from build123d import *

# Parameters (mm, degrees)
SKETCH1_R           = 3.1750000000000016
SKETCH1_R_2         = 3.174999999999998
SKETCH1_R_3         = 3.1749999999999976
BOSS_EXTRUDE1_DEPTH = 5.842
FILLET1_R           = 6.35
FILLET2_R           = 12.7
BOSS_EXTRUDE2_START = -5.842
SKETCH2_R           = 3.3749999999999933
BOSS_EXTRUDE2_DEPTH = 5.842
SKETCH3_R           = 3.174229815615873
CUT_EXTRUDE1_DEPTH  = 74.47150684282778
FILLET3_R           = 6.35
CUT_EXTRUDE2_DEPTH  = 74.47150698753184
FILLET4_R           = 6.35


with BuildPart() as part:
    # Sketch1 → Boss-Extrude1 (new body)
    with BuildSketch(Plane.XY):
        with BuildLine():
            Line((-19.735202783136515, 15.926469991088537), (-23.82219128055887, 21.14411855360569))
            ThreePointArc((-23.82219128055887, 21.14411855360569), (-23.43878883536159, 29.420896018239304), (-15.19702887852625, 30.27262100199607))
            Line((-15.19702887852625, 30.27262100199607), (-1.1351215821202347, 20.490721215283713))
            Line((-1.1351215821202347, 20.490721215283713), (26.98869301069201, 20.49072121528371))
            Line((26.98869301069201, 20.49072121528371), (42.6381003070978, 30.272621001996075))
            ThreePointArc((42.6381003070978, 30.272621001996075), (50.87986026393313, 29.42089601823929), (51.26326270913039, 21.14411855360571))
            Line((51.26326270913039, 21.14411855360571), (47.176274211707955, 15.926469991088574))
            Line((47.176274211707955, 15.926469991088574), (47.176274211707955, 5.491172866054349))
            Line((47.176274211707955, 5.491172866054349), (51.26326270913039, 0.27352430353700524))
            ThreePointArc((51.26326270913039, 0.27352430353700524), (52.26703524751068, -1.5710682312081294), (52.614285714285785, -3.6421785714286505))
            Line((52.614285714285785, -3.6421785714286505), (52.614285714285785, -37.659455709821316))
            Line((52.614285714285785, -37.659455709821316), (-25.173214285713918, -37.659455709821316))
            Line((-25.173214285713918, -37.659455709821316), (-25.173214285713925, -3.6421785714286505))
            ThreePointArc((-25.173214285713925, -3.6421785714286505), (-24.825963818939076, -1.5710682312081503), (-23.822191280558854, 0.27352430353699286))
            Line((-23.822191280558854, 0.27352430353699286), (-19.735202783136522, 5.491172866054132))
            Line((-19.735202783136522, 5.491172866054132), (-19.735202783136515, 15.926469991088537))
        make_face()
        with Locations((-18.823214285714226, 25.059821428571347)):
            Circle(SKETCH1_R, mode=Mode.SUBTRACT)
        with Locations((46.26428571428577, 25.059821428571347)):
            Circle(SKETCH1_R_2, mode=Mode.SUBTRACT)
        with Locations((46.26428571428577, -3.6421785714286505)):
            Circle(SKETCH1_R_3, mode=Mode.SUBTRACT)
        with Locations((-18.823214285713924, -3.6421785714286505)):
            Circle(SKETCH1_R, mode=Mode.SUBTRACT)
    extrude(amount=BOSS_EXTRUDE1_DEPTH)

    # Fillet1
    fillet1_edges = [part.edges().sort_by_distance(p)[0] for p in [
        (47.176274211707955, 15.926469991088574, 2.921),
        (47.176274211707955, 5.491172866054349, 2.921),
        (-19.735202783136522, 5.491172866054132, 2.921),
        (-19.735202783136515, 15.926469991088537, 2.921),
    ]]
    fillet(fillet1_edges, radius=FILLET1_R)

    # Fillet2
    fillet2_edges = [part.edges().sort_by_distance(p)[0] for p in [
        (-1.1351215821202347, 20.490721215283713, 2.921),
        (26.98869301069201, 20.49072121528371, 2.921),
    ]]
    fillet(fillet2_edges, radius=FILLET2_R)

    # Sketch2 → Boss-Extrude2 (add)
    # profile 1 of 2: a face of its own
    with BuildSketch(Plane.XY.offset(5.842).offset(BOSS_EXTRUDE2_START)):
        with BuildLine():
            Line((52.614285714285785, -22.564372384825948), (56.4647972168636, -22.564372384825948))
            ThreePointArc((56.4647972168636, -22.564372384825948), (62.8147972168636, -16.214372384825946), (56.4647972168636, -9.864372384825945))
            Line((56.4647972168636, -9.864372384825945), (51.94643033410118, -0.8074418077232544))
            ThreePointArc((51.94643033410118, -0.8074418077232544), (52.44506715095817, -2.186005219081439), (52.614285714285785, -3.6421785714286505))
            Line((52.614285714285785, -3.6421785714286505), (52.614285714285785, -11.165009933138013))
            Line((52.614285714285785, -11.165009933138013), (52.614285714285785, -21.26373483651388))
            Line((52.614285714285785, -21.26373483651388), (52.614285714285785, -22.564372384825948))
        make_face()
        with Locations((56.4647972168636, -16.214372384825946)):
            Circle(SKETCH2_R, mode=Mode.SUBTRACT)
    # profile 2 of 2: a face of its own
    with BuildSketch(Plane.XY.offset(5.842).offset(BOSS_EXTRUDE2_START)):
        with BuildLine():
            Line((-25.11442078188718, -2.7800760122689354), (-26.085202783136417, -9.864372384825948))
            ThreePointArc((-26.085202783136417, -9.864372384825948), (-32.43520278313642, -16.21437238482595), (-26.085202783136413, -22.56437238482595))
            Line((-26.085202783136417, -22.56437238482595), (-25.17321428571397, -22.56437238482595))
            Line((-25.17321428571397, -22.56437238482595), (-25.17321428571397, -22.49854114294895))
            Line((-25.173214285713975, -22.49854114294895), (-25.173214285713986, -19.254769053504887))
            ThreePointArc((-25.173214285713996, -19.254769053504887), (-29.25943259875229, -16.214372384825957), (-25.17321428571401, -13.173975716147009))
            Line((-25.173214285714007, -13.173975716147009), (-25.17321428571402, -9.930203626702937))
            Line((-25.17321428571402, -9.930203626702937), (-25.173214285714042, -3.6421785714286496))
            ThreePointArc((-25.173214285714042, -3.6421785714286496), (-25.158498859065922, -3.2101260576638357), (-25.11442078188718, -2.7800760122689354))
        make_face()
    extrude(amount=BOSS_EXTRUDE2_DEPTH)

    # Sketch3 → Cut-Extrude1 (cut, through all)
    with BuildSketch(Plane.XY.offset(5.842)):
        with Locations((-26.085202783136417, -16.21437238482595)):
            Circle(SKETCH3_R)
    extrude(amount=-CUT_EXTRUDE1_DEPTH, mode=Mode.SUBTRACT)

    # Fillet3
    fillet3_edges = [part.edges().sort_by_distance(p)[0] for p in [
        (56.4647972168636, -9.864372384825945, 2.921),
        (52.614285714285785, -22.564372384825948, 2.921),
        (-25.17321428571397, -22.56437238482595, 2.921),
        (-26.085202783136417, -9.864372384825948, 2.921),
    ]]
    fillet(fillet3_edges, radius=FILLET3_R)

    # Sketch4 → Cut-Extrude2 (cut, through all)
    with BuildSketch(Plane.XY.offset(5.842)):
        with BuildLine():
            Line((-25.173214285713918, -37.659455709821316), (-12.473214285713917, -37.659455709821316))
            Line((-12.473214285713917, -37.659455709821316), (-27.048811913081487, -23.185421123073148))
            ThreePointArc((-27.048811913081487, -23.185421123073148), (-25.66083613916725, -25.250928515915028), (-25.17321428571392, -27.691219987623278))
            Line((-25.17321428571392, -27.691219987623278), (-25.173214285713918, -37.659455709821316))
        make_face()
        with BuildLine():
            Line((54.888473112152276, -23.796663637650127), (38.326785714286075, -37.659455709821316))
            Line((38.326785714286075, -37.659455709821316), (52.614285714285785, -37.659455709821316))
            Line((52.614285714285785, -37.659455709821316), (52.614285714285785, -28.665981005853762))
            ThreePointArc((52.614285714285785, -28.665981005853762), (53.21085586664066, -25.97887382745055), (54.888473112152276, -23.796663637650127))
        make_face()
    extrude(amount=-CUT_EXTRUDE2_DEPTH, mode=Mode.SUBTRACT)

    # Fillet4
    fillet4_edges = [part.edges().sort_by_distance(p)[0] for p in [
        (-12.473214285713917, -37.659455709821316, 2.921),
        (38.326785714286075, -37.659455709821316, 2.921),
    ]]
    fillet(fillet4_edges, radius=FILLET4_R)


solid = part.part
CAD build for the part. Positions are in the model's coordinates, mm. A direction names the side the tool comes from. Give positions to 0.01 mm unless a question says otherwise; leave off trailing zeros. Loops run counter-clockwise (first coordinate to the right, second up) from the corner with the lowest first, then second, coordinate; pieces in that order, holes last. Notation, with made-up numbers: M -33.75,52.25 L -1.75,52.25 A22 ccw -1.75,86.25 Z; hole C 33,49 d3. An arc over 180 degrees is marked long. One line per question, with ' | ' between items. Start each with the question number.
1. Saw through at B-B on y = 27. Give the cut face in (x, z), plus the area to 3 significant figures.
2. Saw through at C-C on x = 16. Give the cut face in (y, z).
3. Saw through at D-D on z = 2.4. State how many separate pieces and enclosed holes the cut face has, plus the area to 3 significant figures.
4. Probe L1, parallel to X at y = -17, z = 4.1; L2, parallel to X at y = 25.5, z = 0.3; L3, parallel to Y at x = 59.5, z = 1.65. List the from-to ranges inside material, lowest first. Write a range as from..to.
5. Two-plate mould, pull along X, no slides. Class faces 6 (the face through (53.79, -18.27, 2.88)), 7 (the face through (47.514, 5.639, 2.962)), 8 (the face through (15, -3, 0)): pulls with the +X half, pulls with the -X half, needs draft (parallel to the pull), parting line crosses it, or undercut.
6. Saw through at A-A on y = -17.5. Give the cut face in (x, z), plus the area to 3 significant figures.
7. 3-axis set-ups, long thin cutter, end or side, ignore diameter. For faces 1 (the face through (47.6, -29.9, 3)), 2 (the face through (49.293, -2.688, 2.88)), 3 (the face through (-24.68, -1.19, 2.88)), 4 (the face through (49.88, 2.04, 2.88)), 5 (the face through (13, 20.491, 3)): which of +Z, -Z, +X, -X, +Y, -Y reach the whole face in a straight line?
8. Flat gauge pins, fed straight in: pin 1 (1.8 mm diameter, centred on y = 10.5, z = 2.5, fed in from +X); pin 2 (1 mm diameter, centred on x = 44.5, z = 4.5, fed in from +Y); pin 3 (1 mm diameter, centred on x = 46.5, z = 4.5, fed in from -Y). Where does each tip first touch, or does it go through?
Result sheet:
1) outline: M -24.87,0 L -21.34,0 L -21.34,5.84 L -24.87,5.84 Z; M -16.31,0 L -10.49,0 L -10.49,5.84 L -16.31,5.84 Z; M 37.4,0 L 43.75,0 L 43.75,5.84 L 37.4,5.84 Z; M 48.78,0 L 52.31,0 L 52.31,5.84 L 48.78,5.84 Z | area: 112 mm^2
2) outline: M -37.66,0 L 20.49,0 L 20.49,5.84 L -37.66,5.84 Z
3) separate pieces: 1 | enclosed holes: 6 | area: 4,540 mm^2
4) L1: x = -32.39..-29.16, -23.01..53.18, 59.75..62.77 | L2: x = -25.16..-21.97, -15.68..-8.34, 35..43.12, 49.41..52.6 | L3: y = -21.79..-17.69, -14.74..-10.64
5) face 6: undercut | face 7: pulls with the +X half | face 8: needs draft
6) outline: M -32.3,0 L -28.99,0 L -28.99,5.84 L -32.3,5.84 Z; M -23.18,0 L 53.34,0 L 53.34,5.84 L -23.18,5.84 Z; M 59.59,0 L 62.68,0 L 62.68,5.84 L 59.59,5.84 Z | area: 485 mm^2
7) face 1: +Z, -Z, +X, -Y | face 2: +Z, -Z | face 3: +Z, -Z, -X | face 4: +Z, -Z, +X | face 5: +Z, -Z, +Y
8) pin 1: stops at x = 47.18 | pin 2: stops at y = 31.28 | pin 3: stops at y = -31.24
